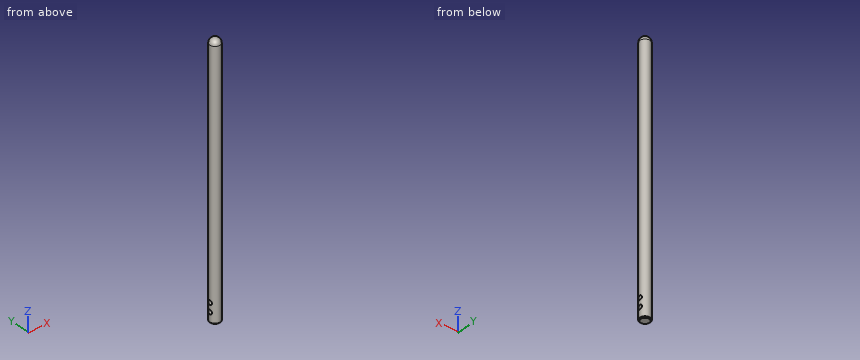
from build123d import *

# Parameters (mm, degrees)
CROQUIS1_R                 = 6
SALIENTE_EXTRUIR1_DEPTH    = 300
REDONDEO1_R                = 6
CORTAR_EXTRUIR1_DEPTH      = 301.11997601
CORTAR_EXTRUIR1_DEPTH_BACK = 301.11997601
CROQUIS2_R                 = 2.5
CHAFL_N1_SIZE              = 1


with BuildPart() as part:
    # Croquis1 → Saliente-Extruir1 (new body)
    with BuildSketch(Plane.XY):
        Circle(CROQUIS1_R)
    extrude(amount=SALIENTE_EXTRUIR1_DEPTH)

    # Redondeo1
    redondeo1_edges = [part.edges().sort_by_distance(p)[0] for p in [
        (-6, 0, 300),
    ]]
    fillet(redondeo1_edges, radius=REDONDEO1_R)

    # Croquis2 → Cortar-Extruir1 (cut, two sides: drawn at the far end of the back side and taken through both)
    with BuildSketch(Plane(origin=(0, 0, 0), x_dir=(0, 0, -1), z_dir=(1, 0, 0)).offset(-CORTAR_EXTRUIR1_DEPTH_BACK)):
        with Locations((-12, 0)):
            Circle(CROQUIS2_R)
        with Locations((-22, 0)):
            Circle(CROQUIS2_R)
    extrude(amount=CORTAR_EXTRUIR1_DEPTH + CORTAR_EXTRUIR1_DEPTH_BACK, mode=Mode.SUBTRACT)

    # Chaflán1
    chafl_n1_edges = [part.edges().sort_by_distance(p)[0] for p in [
        (-6, 0, 0),
    ]]
    chamfer(chafl_n1_edges, length=CHAFL_N1_SIZE)


solid = part.part
Can you work these out from the model? Positions are in its coordinate system, mm. Round coordinates to 2 decimals unless told otherwise and drop trailing zeros. Order: outer loops, then holes, each group sorted by start corner. A loop starts at its lowest first (then second) coordinate and runs counter-clockwise, first axis right, second up. Notation, with made-up numbers: M -29.75,21.5 L -18.75,21.5 A7 cw -18.75,34.5 Z; hole C -17.5,-13 d9. An arc over 180 degrees is marked long. Use a Markdown table: item, result.
1) Imagine slicing it at A-A (y = 0). List the corners of the cut face in (x, z) for me, then the cut area to 3 significant figures.
Geometry says:
| item | result |
|---|---|
| outline | M -6,1 L -5,0 L 5,0 L 6,1 L 6,9.5 L -6,9.5 Z; M -6,14.5 L 6,14.5 L 6,19.5 L -6,19.5 Z; M -6,24.5 L 6,24.5 L 6,294 A6 ccw -6,294 Z |
| area | 3,460 mm² |
2) Imagine slicing it at B-B (x = 0). List the corners of the cut face in (y, z) for me.
Geometry says:
| item | result |
|---|---|
| outline | M -6,1 L -5,0 L 5,0 L 6,1 L 6,294 A6 ccw -6,294 Z; hole C 0,12 d5; hole C 0,22 d5 |
3) I'm going to push flat-ended pins straight in: P1, Ø1.5, axis at y = 3, z = 112.5, coming from the -X side; P2, Ø3, axis at x = -4, y = 2.5, coming from the +Z side; P3, Ø4, axis at y = 5, z = 87, coming from the -X side. Where does each tip first touch, or does it pass through?
Geometry says:
| item | result |
|---|---|
| P1 | stops at x = -5.56 |
| P2 | stops at z = 299.06 |
| P3 | stops at x = -5.2 |
4) Imagine slicing it at D-D (z = 113). List the corners of the cut face in (x, y) for me.
Geometry says:
| item | result |
|---|---|
| outline | C 0,0 d12 |
5) Imagine slicing it at C-C (z = 12). List the corners of the cut face in (x, y) for me, then the cut area to 3 significant figures.
Geometry says:
| item | result |
|---|---|
| outline | M -5.45,-2.5 A6 ccw 5.45,-2.5 Z; M -5.45,2.5 L 5.45,2.5 A6 ccw Z |
| area | 54.9 mm² |
6) If I drill on line 1 along Z through (x, y) = (0.25, 0); line 2 along Y through (x, z) = (3.25, 12); line 3 along Z through (x, y) = (4.25, -1.25), over which ranges is the centre line in solid material (lowest first)?
Geometry says:
| item | result |
|---|---|
| line 1 | z = 0 to 9.5, 14.5 to 19.5, 24.5 to 299.99 |
| line 2 | y = -5.04 to -2.5, 2.5 to 5.04 |
| line 3 | z = 0 to 9.83, 14.17 to 19.83, 24.17 to 298.05 |
